Geometry check sheet. Reference: the model listing, model coordinates, mm. Round coordinates to 2 decimals unless told otherwise and drop trailing zeros. Order: outer loops, then holes, each group sorted by start corner. A loop starts at its lowest first (then second) coordinate and runs counter-clockwise, first axis right, second up.
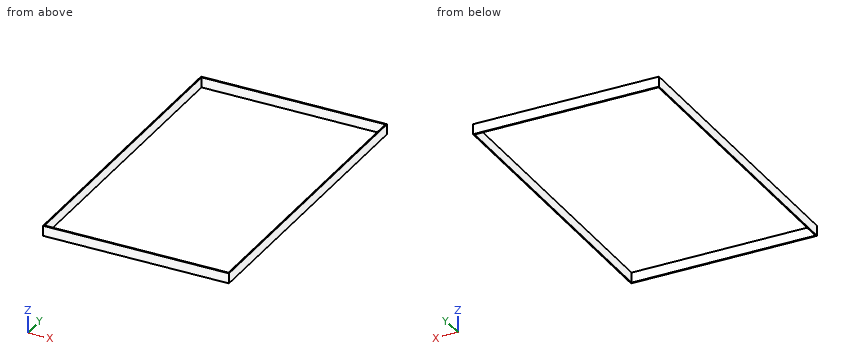
```python
from build123d import *

# Parameters (mm, degrees)
ESBO_O1_W                = 182
ESBO_O1_H                = 297
ESBO_O1_W_2              = 180
ESBO_O1_H_2              = 295
RESSALTO_EXTRUS_O1_DEPTH = 10


with BuildPart() as part:
    # Esboço1 → Ressalto-extrusão1 (new body)
    with BuildSketch(Plane.XY):
        Rectangle(ESBO_O1_W, ESBO_O1_H)
        Rectangle(ESBO_O1_W_2, ESBO_O1_H_2, mode=Mode.SUBTRACT)
    extrude(amount=RESSALTO_EXTRUS_O1_DEPTH)


solid = part.part
```
(1) Sectioned sample at A-A, the plane z = 7.25. Record the cut outline in (x, y).
Returned:
outline: (-91, -148.5) - (91, -148.5) - (91, 148.5) - (-91, 148.5) - close; hole (-90, -147.5) - (90, -147.5) - (90, 147.5) - (-90, 147.5) - close
(2) Sectioned sample at B-B, the plane y = 42. Record the cut outline in (x, z).
Returned:
outline: (-91, 0) - (-90, 0) - (-90, 10) - (-91, 10) - close; (90, 0) - (91, 0) - (91, 10) - (90, 10) - close
(3) Material ranges on line 1 (Y direction, x = 22.5, z = 8.5); line 2 (X direction, y = -121, z = 2), recorded low to high.
Returned:
line 1: y = -148.5 to -147.5, 147.5 to 148.5
line 2: x = -91 to -90, 90 to 91
(4) Sectioned sample at C-C, the plane x = -32. Record the cut outline in (y, z), and give its area (3 significant figures).
Returned:
outline: (-148.5, 0) - (-147.5, 0) - (-147.5, 10) - (-148.5, 10) - close; (147.5, 0) - (148.5, 0) - (148.5, 10) - (147.5, 10) - close
area: 20.0 mm2
